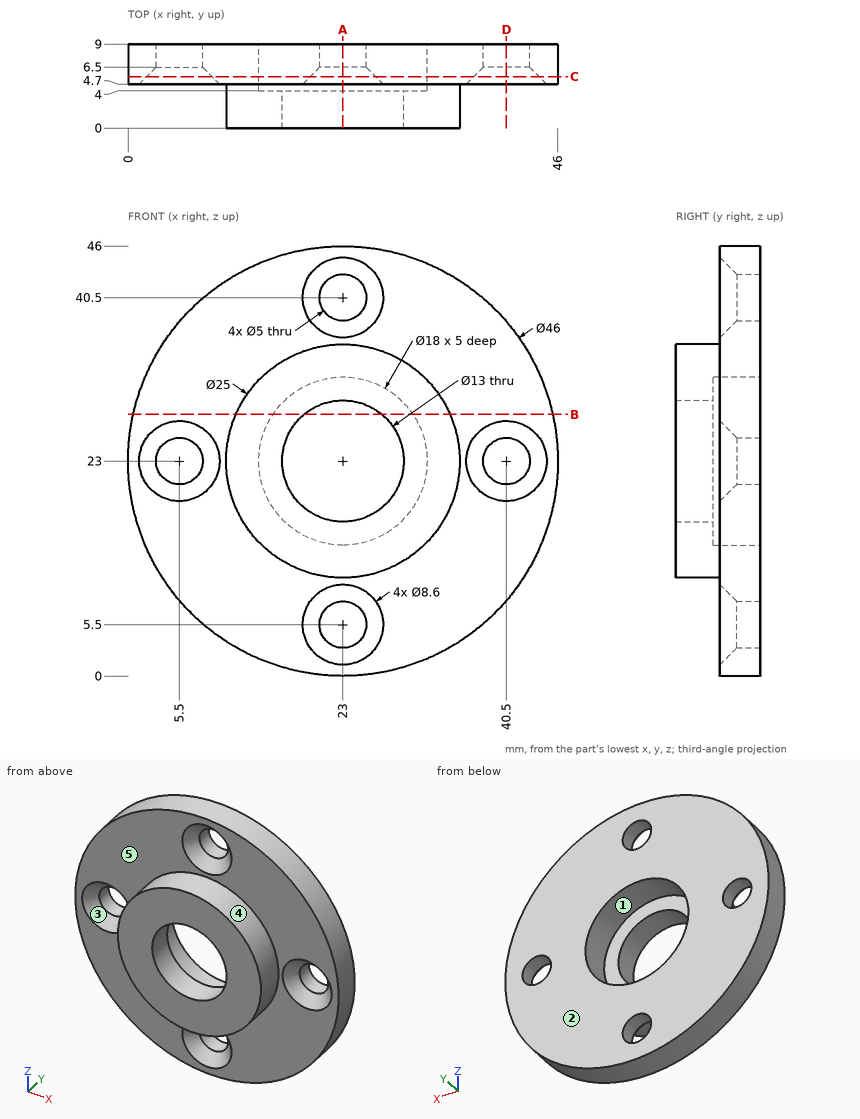
Check sheet for the drawn part. Datum: minimum x, y, z corner. Units: mm. A direction names the side the tool comes from. Give positions to 0.01 mm unless a question says otherwise; leave off trailing zeros. Loops run counter-clockwise (first coordinate to the right, second up) from the corner with the lowest first, then second, coordinate; pieces in that order, holes last. Notation, with made-up numbers: M -21,-32 L 8,-32 A21 cw 8,-2 Z; hole C 82.25,-22.75 d10. An arc over 180 degrees is marked long. Answer as CSV lines item,"result".
Item 1: Draft check along Z on the marked faces 3, 4 and 5. Enter one of: pulls with the +Z half, pulls with the -Z half, needs draft (parallel to the pull), parting line crosses it, or undercut.
Reply:
face 3,"undercut"
face 4,"parting line crosses it"
face 5,"needs draft"
Item 2: Sectioned sample at C-C, the plane y = 5.5. Enter the section's corners in (x, z).
Reply:
outline,"C 23,23 d46; hole C 5.5,23 d7; hole C 23,23 d18; hole C 23,5.5 d7; hole C 23,40.5 d7; hole C 40.5,23 d7"
Item 3: Set-up check for the marked faces 1 and 2: record each of +Z, -Z, +X, -X, +Y, -Y from which the full face is reachable in a straight line by a thin tool's end or side.
Reply:
face 1,"+Y"
face 2,"+Z, -Z, +X, -X, +Y"
Item 4: Sectioned sample at D-D, the plane x = 40.5. Enter the section's corners in (y, z), then the cut area to 3 significant figures.
Reply:
outline,"M 4.7,8.08 L 9,8.08 L 9,20.5 L 6.5,20.5 L 4.7,18.7 Z; M 4.7,27.3 L 6.5,25.5 L 9,25.5 L 9,37.92 L 4.7,37.92 Z"
area,"104 mm^2"
Item 5: Sectioned sample at A-A, the plane x = 23. Enter the section's corners in (y, z).
Reply:
outline,"M 0,10.5 L 4.7,10.5 L 4.7,9.8 L 6.5,8 L 9,8 L 9,14 L 4,14 L 4,16.5 L 0,16.5 Z; M 0,29.5 L 4,29.5 L 4,32 L 9,32 L 9,38 L 6.5,38 L 4.7,36.2 L 4.7,35.5 L 0,35.5 Z; M 4.7,0 L 9,0 L 9,3 L 6.5,3 L 4.7,1.2 Z; M 4.7,44.8 L 6.5,43 L 9,43 L 9,46 L 4.7,46 Z"
Item 6: Sectioned sample at B-B, the plane z = 28. Enter the section's corners in (x, y).
Reply:
outline,"M 0.55,4.7 L 11.54,4.7 L 11.54,0 L 18.85,0 L 18.85,4 L 15.52,4 L 15.52,9 L 0.55,9 Z; M 27.15,0 L 34.46,0 L 34.46,4.7 L 45.45,4.7 L 45.45,9 L 30.48,9 L 30.48,4 L 27.15,4 Z"
Item 7: Scan lines: L1, parallel to X at y = 7.2, z = 23; L2, parallel to Z at x = 23, y = 2.05; L3, parallel to Z at x = 25, y = 8. Record each from-to range of solid material in increasing order.
Reply:
L1,"0 to 3, 8 to 14, 32 to 38, 43 to 46"
L2,"10.5 to 16.5, 29.5 to 35.5"
L3,"0.09 to 4, 7 to 14.23, 31.77 to 39, 42 to 45.91"
Item 8: Depth check by flat-ended pin: pin 1 Ø1 at (y, z) = (4.5, 10.5) entering from +X; pin 2 Ø4 at (x, y) = (34, 5.5) entering from +Z; pin 3 Ø3 at (x, z) = (23, 5.5) entering from -Y; pin 4 Ø4 at (y, z) = (7, 39.5) entering from -X. Enter the tip coordinate at first touch or a pass-through.
Reply:
pin 1,"x = 42.6"
pin 2,"z = 44.17"
pin 3,"through"
pin 4,"x = 5.15"
